Work out the finished part from the listing and answer in its coordinate system (mm). Face numbers are marked on the shaded views. A direction names the side the tool comes from. Give positions to 0.01 mm unless a question says otherwise; leave off trailing zeros. Write each loop counter-clockwise with the first axis right and the second up, starting at its lowest first coordinate (ties: lowest second). Pieces come first, ordered by that corner, then holes. Notation, with made-up numbers: (-26, 88) -> (17, 88) arc R29 ccw to (17, 125) -> close; hole circle Ø2 at (-16, 47.5). An arc over 180 degrees is marked (long way). Use a Markdown table: item, result. Add a question column.
Q1. Section C-C, the plane y = -6.5 is taken. Give the vertices of the cut face in (x, z).
Q2. Section B-B, the plane x = -42.5 is taken. State how many separate pieces and enclosed holes the cut face has, plus the area to 3 significant figures.
Q3. Section D-D, the plane z = -78 is taken. Give the vertices of the cut face in (x, y).
Q4. Section A-A, the plane y = -19 is taken. Give the vertices of the cut face in (x, z).
Q5. For the marked faces 1 and 2, determine the directions among +Z, -Z, +X, -X, +Y, -Y from which every point of the face is accessible in a straight line to the end or side of a thin tool.
Q6. Each of these flat-tipped pins is pushed along its axis until it touches: pin 1 Ø1.5 at (y, z) = (-16, 62) entering from -X; pin 2 Ø3 at (x, z) = (66, -15.5) entering from -Y. Where does it stop, or does it pass through?
Q7. Consider line 1 (Y direction, x = -2, z = 4); line 2 (Z direction, x = -14, y = -12); line 3 (Z direction, x = -69, y = 0). Determine where each line is inside the solid, lowest interval first.
from build123d import *

# Parameters (mm, degrees)
BOSS_EXTRUDE2_DEPTH  = 1
MOTOR_SPACING_W      = 153.743038476
MOTOR_SPACING_H      = 35
BOSS_EXTRUDE6_DEPTH  = 2
FILLET4_START        = -1
FILLET4_DEPTH        = 2
FILLET6_R            = 35
FILLET7_R            = 1
PIR_ULTRA_W          = 45
PIR_ULTRA_H          = 5
BOSS_EXTRUDE10_DEPTH = 22
CUT_EXTRUDE4_DEPTH   = 22
SKETCH4_R            = 4
CUT_EXTRUDE5_DEPTH   = 10


with BuildPart() as part:
    # Top_lay → Boss-Extrude2 (new, symmetric)
    with BuildSketch(Plane(origin=(0, 0, 0), x_dir=(1, 0, 0), z_dir=(0, 1, 0))):
        with BuildLine():
            ThreePointArc((27.849459475, -85.582752976), (0, 90), (-27.849459475, -85.582752976))
            ThreePointArc((-27.849459475, -85.582752976), (-14.598708504, -78.839227398), (0, -76.022270085))
            ThreePointArc((0, -76.022270085), (14.598708504, -78.839227398), (27.849459475, -85.582752976))
        make_face()
    extrude(amount=BOSS_EXTRUDE2_DEPTH, both=True)

    # Motor_Spacing → Boss-Extrude6 (add)
    with BuildSketch(Plane(origin=(0, 1, 0), x_dir=(1, 0, 0), z_dir=(0, 1, 0))):
        with Locations((0, 63.828780022)):
            Rectangle(MOTOR_SPACING_W, MOTOR_SPACING_H)
    extrude(amount=-BOSS_EXTRUDE6_DEPTH)

    # Fillet4: read off the stored shape, not the designer's step
    # Fillet4 outline → Fillet4 (add)
    with BuildSketch(Plane(origin=(0, 0, 0), x_dir=(1, 0, 0), z_dir=(0, 1, 0)).offset(FILLET4_START)):
        with BuildLine():
            ThreePointArc((-38.543865143, 81.328780022), (-25.041990736, 86.445929343), (-10.895560747, 89.338047639))
            ThreePointArc((-10.895560747, 89.338047639), (-43.882431037, 85.324278863), (-76.871519238, 81.328780022))
            Line((-76.871519238, 81.328780022), (-38.543865143, 81.328780022))
        make_face()
        with BuildLine():
            ThreePointArc((76.871519238, 81.328780022), (43.882431037, 85.324278863), (10.895560747, 89.338047639))
            ThreePointArc((10.895560747, 89.338047639), (25.041990736, 86.445929343), (38.543865143, 81.328780022))
            Line((38.543865143, 81.328780022), (76.871519238, 81.328780022))
        make_face()
    extrude(amount=FILLET4_DEPTH)

    # Fillet6
    fillet6_edges = [part.edges().sort_by_distance(p)[0] for p in [
        (0, 0, 76.022270085),
    ]]
    fillet(fillet6_edges, radius=FILLET6_R)

    # Fillet7
    fillet7_edges = [part.edges().sort_by_distance(p)[0] for p in [
        (84.399606762, 1, 31.252301969),
        (84.399606762, -1, 31.252301969),
    ]]
    fillet(fillet7_edges, radius=FILLET7_R - 0.0001)  # a hair under: the kernel refuses the full size

    # PIR_ULTRA → Boss-Extrude10 (add)
    with BuildSketch(Plane.XZ.offset(1)):
        with Locations((0, 61.550217006)):
            Rectangle(PIR_ULTRA_W, PIR_ULTRA_H)
    extrude(amount=BOSS_EXTRUDE10_DEPTH)

    # Sketch3 → Cut-Extrude4 (cut)
    with BuildSketch(Plane.XY.offset(64.050217006)):
        with BuildLine():
            Line((-7.578758104, -23), (-7.421241896, -23))
            ThreePointArc((-7.421241896, -23), (-14.921241896, -15.5), (-22.421241896, -23))
            Line((-22.421241896, -23), (-7.578758104, -23))
        make_face()
        with BuildLine():
            ThreePointArc((22.421241896, -23), (14.921241896, -15.5), (7.421241896, -23))
            Line((7.421241896, -23), (22.421241896, -23))
        make_face()
    extrude(amount=-CUT_EXTRUDE4_DEPTH, mode=Mode.SUBTRACT)

    # Sketch4 → Cut-Extrude5 (cut)
    with BuildSketch(Plane.XZ.offset(1)):
        with Locations(Location((-59.5, -67.926375212, 0), (0, 0, 270))):
            Circle(SKETCH4_R)
        with Locations(Location((-25.5, -67.926375212, 0), (0, 0, 270))):
            Circle(SKETCH4_R)
        with Locations(Location((-42.5, -67.926375212, 0), (0, 0, 270))):
            Circle(SKETCH4_R)
        with Locations(Location((-8.5, -67.926375212, 0), (0, 0, 270))):
            Circle(SKETCH4_R)
        with Locations(Location((8.5, -67.926375212, 0), (0, 0, 270))):
            Circle(SKETCH4_R)
        with Locations(Location((25.5, -67.926375212, 0), (0, 0, 270))):
            Circle(SKETCH4_R)
        with Locations(Location((42.5, -67.926375212, 0), (0, 0, 270))):
            Circle(SKETCH4_R)
        with Locations(Location((59.5, -67.926375212, 0), (0, 0, 270))):
            Circle(SKETCH4_R)
        with Locations(Location((-59.5, -52.926375212, 0), (0, 0, 270))):
            Circle(SKETCH4_R)
        with Locations(Location((25.5, -52.926375212, 0), (0, 0, 270))):
            Circle(SKETCH4_R)
        with Locations(Location((-42.5, -52.926375212, 0), (0, 0, 270))):
            Circle(SKETCH4_R)
        with Locations(Location((-25.5, -52.926375212, 0), (0, 0, 270))):
            Circle(SKETCH4_R)
        with Locations(Location((8.5, -52.926375212, 0), (0, 0, 270))):
            Circle(SKETCH4_R)
        with Locations(Location((42.5, -52.926375212, 0), (0, 0, 270))):
            Circle(SKETCH4_R)
        with Locations(Location((59.5, -52.926375212, 0), (0, 0, 270))):
            Circle(SKETCH4_R)
        with Locations(Location((-8.5, -52.926375212, 0), (0, 0, 270))):
            Circle(SKETCH4_R)
        with Locations(Location((-59.5, -37.926375212, 0), (0, 0, 270))):
            Circle(SKETCH4_R)
        with Locations(Location((25.5, -37.926375212, 0), (0, 0, 270))):
            Circle(SKETCH4_R)
        with Locations(Location((-42.5, -37.926375212, 0), (0, 0, 270))):
            Circle(SKETCH4_R)
        with Locations(Location((-25.5, -37.926375212, 0), (0, 0, 270))):
            Circle(SKETCH4_R)
        with Locations(Location((8.5, -37.926375212, 0), (0, 0, 270))):
            Circle(SKETCH4_R)
        with Locations(Location((42.5, -37.926375212, 0), (0, 0, 270))):
            Circle(SKETCH4_R)
        with Locations(Location((59.5, -37.926375212, 0), (0, 0, 270))):
            Circle(SKETCH4_R)
        with Locations(Location((-8.5, -37.926375212, 0), (0, 0, 270))):
            Circle(SKETCH4_R)
        with Locations(Location((-59.5, -22.926375212, 0), (0, 0, 270))):
            Circle(SKETCH4_R)
        with Locations(Location((25.5, -22.926375212, 0), (0, 0, 270))):
            Circle(SKETCH4_R)
        with Locations(Location((-42.5, -22.926375212, 0), (0, 0, 270))):
            Circle(SKETCH4_R)
        with Locations(Location((-25.5, -22.926375212, 0), (0, 0, 270))):
            Circle(SKETCH4_R)
        with Locations(Location((8.5, -22.926375212, 0), (0, 0, 270))):
            Circle(SKETCH4_R)
        with Locations(Location((42.5, -22.926375212, 0), (0, 0, 270))):
            Circle(SKETCH4_R)
        with Locations(Location((59.5, -22.926375212, 0), (0, 0, 270))):
            Circle(SKETCH4_R)
        with Locations(Location((-8.5, -22.926375212, 0), (0, 0, 270))):
            Circle(SKETCH4_R)
        with Locations(Location((-59.5, -7.926375212, 0), (0, 0, 270))):
            Circle(SKETCH4_R)
        with Locations(Location((25.5, -7.926375212, 0), (0, 0, 270))):
            Circle(SKETCH4_R)
        with Locations(Location((-42.5, -7.926375212, 0), (0, 0, 270))):
            Circle(SKETCH4_R)
        with Locations(Location((-25.5, -7.926375212, 0), (0, 0, 270))):
            Circle(SKETCH4_R)
        with Locations(Location((8.5, -7.926375212, 0), (0, 0, 270))):
            Circle(SKETCH4_R)
        with Locations(Location((42.5, -7.926375212, 0), (0, 0, 270))):
            Circle(SKETCH4_R)
        with Locations(Location((59.5, -7.926375212, 0), (0, 0, 270))):
            Circle(SKETCH4_R)
        with Locations(Location((-8.5, -7.926375212, 0), (0, 0, 270))):
            Circle(SKETCH4_R)
        with Locations(Location((-59.5, 7.073624788, 0), (0, 0, 270))):
            Circle(SKETCH4_R)
        with Locations(Location((25.5, 7.073624788, 0), (0, 0, 270))):
            Circle(SKETCH4_R)
        with Locations(Location((-42.5, 7.073624788, 0), (0, 0, 270))):
            Circle(SKETCH4_R)
        with Locations(Location((-25.5, 7.073624788, 0), (0, 0, 270))):
            Circle(SKETCH4_R)
        with Locations(Location((8.5, 7.073624788, 0), (0, 0, 270))):
            Circle(SKETCH4_R)
        with Locations(Location((42.5, 7.073624788, 0), (0, 0, 270))):
            Circle(SKETCH4_R)
        with Locations(Location((59.5, 7.073624788, 0), (0, 0, 270))):
            Circle(SKETCH4_R)
        with Locations(Location((-8.5, 7.073624788, 0), (0, 0, 270))):
            Circle(SKETCH4_R)
        with Locations(Location((-59.5, 22.073624788, 0), (0, 0, 270))):
            Circle(SKETCH4_R)
        with Locations(Location((25.5, 22.073624788, 0), (0, 0, 270))):
            Circle(SKETCH4_R)
        with Locations(Location((-42.5, 22.073624788, 0), (0, 0, 270))):
            Circle(SKETCH4_R)
        with Locations(Location((-25.5, 22.073624788, 0), (0, 0, 270))):
            Circle(SKETCH4_R)
        with Locations(Location((8.5, 22.073624788, 0), (0, 0, 270))):
            Circle(SKETCH4_R)
        with Locations(Location((42.5, 22.073624788, 0), (0, 0, 270))):
            Circle(SKETCH4_R)
        with Locations(Location((59.5, 22.073624788, 0), (0, 0, 270))):
            Circle(SKETCH4_R)
        with Locations(Location((-8.5, 22.073624788, 0), (0, 0, 270))):
            Circle(SKETCH4_R)
        with Locations(Location((-59.5, 37.073624788, 0), (0, 0, 270))):
            Circle(SKETCH4_R)
        with Locations(Location((25.5, 37.073624788, 0), (0, 0, 270))):
            Circle(SKETCH4_R)
        with Locations(Location((-42.5, 37.073624788, 0), (0, 0, 270))):
            Circle(SKETCH4_R)
        with Locations(Location((-25.5, 37.073624788, 0), (0, 0, 270))):
            Circle(SKETCH4_R)
        with Locations(Location((8.5, 37.073624788, 0), (0, 0, 270))):
            Circle(SKETCH4_R)
        with Locations(Location((42.5, 37.073624788, 0), (0, 0, 270))):
            Circle(SKETCH4_R)
        with Locations(Location((59.5, 37.073624788, 0), (0, 0, 270))):
            Circle(SKETCH4_R)
        with Locations(Location((-8.5, 37.073624788, 0), (0, 0, 270))):
            Circle(SKETCH4_R)
    extrude(amount=-CUT_EXTRUDE5_DEPTH, mode=Mode.SUBTRACT)


solid = part.part
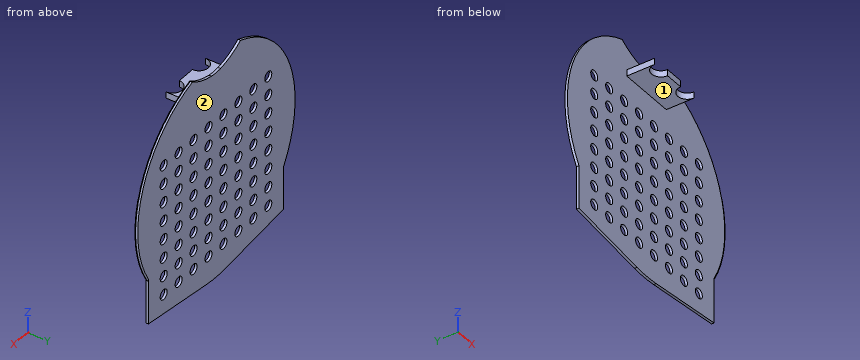
Result set:
| question | item | result |
|---|---|---|
| 1 | outline | (-22.5, 59.05) -> (22.5, 59.05) -> (22.5, 64.05) -> (-22.5, 64.05) -> close |
| 2 | separate pieces | 9 |
| 2 | enclosed holes | 0 |
| 2 | area | 202 mm2 |
| 3 | outline | (-76.87, -1) -> (76.87, -1) -> (76.87, 1) -> (-76.87, 1) -> close |
| 4 | outline | (-22.5, 59.05) -> (-21.27, 59.05) -> (-21.27, 64.05) -> (-22.5, 64.05) -> close; (-8.58, 59.05) -> (8.58, 59.05) -> (8.58, 64.05) -> (-8.58, 64.05) -> close; (21.27, 59.05) -> (22.5, 59.05) -> (22.5, 64.05) -> (21.27, 64.05) -> close |
| 5 | face 1 | -Z, +X, -X, -Y |
| 5 | face 2 | +Z, -Z, +X, -X, +Y |
| 6 | pin 1 | stops at x = -22.5 |
| 6 | pin 2 | stops at y = -1 |
| 7 | line 1 | y = -1 to 1 |
| 7 | line 2 | z = 59.05 to 64.05 |
| 7 | line 3 | z = -82.28 to 57.78 |
